Check sheet for the modelled part. Datum: model origin and axes. Units: mm. A direction names the side the tool comes from. Give positions to 0.01 mm unless a question says otherwise; leave off trailing zeros. Loops run counter-clockwise (first coordinate to the right, second up) from the corner with the lowest first, then second, coordinate; pieces in that order, holes last. Notation, with made-up numbers: (18.25, 80) - (41.25, 80) arc R20 ccw to (41.25, 84) - close; hole circle Ø8 at (21, 59.5). An arc over 180 degrees is marked (long way). Use CSV: the item, a comma, the result in double quotes.
from build123d import *

# Parameters (mm, degrees)
F0_W      = 60
F0_H      = 40
F0_R      = 6
F1_DEPTH  = 6
F2_W      = 8
F2_H      = 10
F3_DEPTH  = 60
F4_R      = 2
F5_DEPTH  = 10
F6_R      = 1.75
F7_DEPTH  = 10
F8_R      = 7.5
F9_DEPTH  = 0.8
F10_R     = 7.5
F11_DEPTH = 0.8
F12_W     = 20
F12_H     = 24
F13_DEPTH = 25
F14_R     = 3
F15_R     = 4
F16_DEPTH = 40.001


with BuildPart() as f1:
    # F0 (on Top) → F1 (new body, symmetric)
    with BuildSketch(Plane.XY):
        Rectangle(F0_W, F0_H)
        Circle(F0_R, mode=Mode.SUBTRACT)
    extrude(amount=F1_DEPTH, both=True)

    # F2 (on face) → F3 (join, through all)
    with BuildSketch(Plane.YZ.offset(30)):
        with Locations((16, 11)):
            Rectangle(F2_W, F2_H)
        with Locations((-16, 11)):
            Rectangle(F2_W, F2_H)
    extrude(amount=-F3_DEPTH)

    # F4 (on face) → F5 (cut)
    with BuildSketch(Plane(origin=(0, 20, 0), x_dir=(-1, 0, 0), z_dir=(0, 1, 0))):
        with Locations((16, 9)):
            Circle(F4_R)
        with Locations((-16, 9)):
            Circle(F4_R)
        with Locations((16, 1)):
            Circle(F4_R)
        with Locations((-16, 1)):
            Circle(F4_R)
    extrude(amount=-F5_DEPTH, mode=Mode.SUBTRACT)

    # F6 (on face) → F7 (cut)
    with BuildSketch(Plane.XZ.offset(20)):
        with Locations((16, 9)):
            Circle(F6_R)
        with Locations((-16, 9)):
            Circle(F6_R)
        with Locations((16, 1)):
            Circle(F6_R)
        with Locations((-16, 1)):
            Circle(F6_R)
    extrude(amount=-F7_DEPTH, mode=Mode.SUBTRACT)

    # F8 (on face) → F9 (cut)
    with BuildSketch(Plane.XY.offset(6)):
        Circle(F8_R)
    extrude(amount=-F9_DEPTH, mode=Mode.SUBTRACT)

    # F10 (on face) → F11 (cut)
    with BuildSketch(Plane(origin=(0, 0, -6), x_dir=(1, 0, 0), z_dir=(0, 0, -1))):
        Circle(F10_R)
    extrude(amount=-F11_DEPTH, mode=Mode.SUBTRACT)

    # F12 (on face) → F13 (cut)
    with BuildSketch(Plane.XY.offset(6)):
        with Locations((20, 0)):
            Rectangle(F12_W, F12_H)
        with Locations((-20, 0)):
            Rectangle(F12_W, F12_H)
    extrude(amount=-F13_DEPTH, mode=Mode.SUBTRACT)

    # F14
    f14_edges = [f1.edges().sort_by_distance(p)[0] for p in [
        (-10, 12, 0),
        (10, 12, 0),
        (10, -12, 0),
        (-10, -12, 0),
    ]]
    fillet(f14_edges, radius=F14_R)

    # F15 (on face) → F16 (cut, through all)
    with BuildSketch(Plane(origin=(0, 20, 0), x_dir=(-1, 0, 0), z_dir=(0, 1, 0))):
        with Locations((24, 5)):
            Circle(F15_R)
        with Locations((-24, 5)):
            Circle(F15_R)
    extrude(amount=-F16_DEPTH, mode=Mode.SUBTRACT)


solid = f1.part
1. Sectioned sample at D-D, the plane x = -24. Record the boundary of the cut face in (y, z).
Completed:
outline,"(-20, -6) - (-12, -6) - (-12, 1) - (-20, 1) - close; (-20, 9) - (-12, 9) - (-12, 16) - (-20, 16) - close; (12, -6) - (20, -6) - (20, 1) - (12, 1) - close; (12, 9) - (20, 9) - (20, 16) - (12, 16) - close"
2. Release check for a two-part mould opening along Z. For faces 1 (the face through (-14.4, 16.1, -0.2)), 2 (the face through (-7.493, -0.33, -5.606)), 3 (the face through (2, -6, -5.2)), 4 (the face through (2, 6, 5.2)) record: released by +Z, released by -Z, zero draft, split by the parting line, or undercut.
Completed:
face 1,"undercut"
face 2,"zero draft"
face 3,"released by -Z"
face 4,"released by +Z"
3. Set-up check for faces 5 (the face through (10, 0, 0)), 6 (the face through (-30, -16, 5)), 7 (the face through (-10.9, -11.14, -0.08)), 8 (the face through (17.6, 16.1, -0.2)), 9 (the face through (27.2, 16.1, 2.6)): record each of +Z, -Z, +X, -X, +Y, -Y from which the full face is reachable in a straight line by a thin tool's end or side.
Completed:
face 5,"+Z, -Z, +X"
face 6,"+Z, -Z, -X, +Y, -Y"
face 7,"+Z, -Z, -X"
face 8,"+Y"
face 9,"+Y, -Y"
4. Sectioned sample at A-A, the plane x = -16. Record the boundary of the cut face in (y, z), and give its area (3 significant figures).
Completed:
outline,"(-20, -6) - (-12, -6) - (-12, -0.75) - (-20, -0.75) - close; (-20, 2.75) - (-12, 2.75) - (-12, 7.25) - (-20, 7.25) - close; (-20, 10.75) - (-12, 10.75) - (-12, 16) - (-20, 16) - close; (12, -6) - (20, -6) - (20, -1) - (12, -1) - close; (12, 3) - (20, 3) - (20, 7) - (12, 7) - close; (12, 11) - (20, 11) - (20, 16) - (12, 16) - close"
area,"232 mm²"
5. Sectioned sample at C-C, the plane y = 17.5. Record the boundary of the cut face in (x, z).
Completed:
outline,"(-30, -6) - (30, -6) - (30, 16) - (-30, 16) - close; hole circle Ø8 at (-24, 5); hole circle Ø4 at (-16, 1); hole circle Ø4 at (-16, 9); hole circle Ø4 at (16, 1); hole circle Ø4 at (16, 9); hole circle Ø8 at (24, 5)"
6. Scan lines: line 1 along Z through (x, y) = (-16, 17); line 2 along Y through (x, z) = (-23, 10); line 3 along Y through (x, z) = (0, -2). Record each from-to range of solid material in increasing order.
Completed:
line 1,"z = -6 to -1, 3 to 7, 11 to 16"
line 2,"y = -20 to -12, 12 to 20"
line 3,"y = -20 to -6, 6 to 20"
7. Sectioned sample at B-B, the plane z = 13.5. Record the boundary of the cut face in (x, y).
Completed:
outline,"(-30, -20) - (30, -20) - (30, -12) - (-30, -12) - close; (-30, 12) - (30, 12) - (30, 20) - (-30, 20) - close"
8. Go/stop test with flat-tipped pins: pin 1 Ø17 at (x, y) = (0, 0) entering from +Z; pin 2 Ø5 at (x, z) = (-16, 1) entering from +Y; pin 3 Ø3 at (y, z) = (-7, 7) entering from +X; pin 4 Ø1 at (y, z) = (9.5, 0.5) entering from +X. Record where each tip stops, or that it passes through.
Completed:
pin 1,"stops at z = 6"
pin 2,"stops at y = 20"
pin 3,"stops at x = 10"
pin 4,"stops at x = 10.17"
